Build history of the part. All positions in model axes, mm. Give positions to 0.01 mm unless a question says otherwise; leave off trailing zeros. Loops run counter-clockwise (first coordinate to the right, second up) from the corner with the lowest first, then second, coordinate; pieces in that order, holes last. Notation, with made-up numbers: M 85.25,-27.75 L 143.25,-27.75 A17 cw 143.25,-23.75 Z; hole C 21,-19 d3. An arc over 180 degrees is marked long. Answer as a JSON object with one key per item and string values. Group by question number.
1. Slice it at A-A (y = 25.4). List the corners of the cut face in (x, z).
2. Mould opens along Y. For faces 1 (the face through (0, 1, 6.35)), 2 (the face through (-23.41, 61.62, 3.22)), 3 (the face through (-13.5, 56.4, 3.2)) say: released by +Y, released by -Y, zero draft, split by the parting line, or undercut.
3. Slice it at C-C (x = 12.7). List the corners of the cut face in (y, z).
4. Drop a flat-ended pin along its axis: pin 1 Ø3 at (x, y) = (-12.7, 53.975) entering from -Z. Give the stop position or say it passes through.
5. Drill centre lines: line 1 along X through (y, z) = (-38.1, 3.75); line 2 along Y through (x, z) = (-12.7, 3.5); line 3 along Y through (x, z) = (13, 6). Where is each one in solid material? Low to high. Write a range as [from, to].
6. Slice it at B-B (z = 1). List the corners of the cut face in (x, y) (3 decimals), then the cut area to 3 significant figures.
Autodesk Inventor part; units mm, degrees
ref_plane "YZ Plane" through (0, 0, 0) normal (1, 0, 0) x (0, 1, 0)
ref_plane "XZ Plane" through (0, 0, 0) normal (0, 1, 0) x (-1, 0, 0)
ref_plane "XY Plane" through (0, 0, 0) normal (0, 0, 1) x (1, 0, 0)
sketch "Sketch1" plane through (0, 0, 0) normal (0, 0, 1) x (1, 0, 0)
  line L0 (25.4, -63.5) -> (-25.4, -63.5)
  line L1 (-25.4, -63.5) -> (-25.4, 63.5)
  line L2 (-25.4, 63.5) -> (25.4, 63.5)
  line L3 (25.4, 63.5) -> (25.4, -63.5)
  line L4 (25.4, -63.5) -> (-25.4, 63.5) construction
  line L5 (-25.4, -63.5) -> (25.4, 63.5) construction
  line L6 (-12.7, 53.975) -> (12.7, 53.975) construction
  point P0 (0, 0)
  point P1 (-12.7, 25.4)
  point P2 (12.7, 25.4)
  point P3 (12.7, -38.1)
  point P4 (-12.7, -38.1)
  point P5 (0, 53.975)
  point P6 (0, 63.5)
  dimension "d0" = 50.8
  dimension "d1" = 127
  dimension "d2" = 9.525
  dimension "d3" = 25.4
  dimension "d4" = 38.1
  dimension "d5" = 63.5
extrude "Extrusion1" add sketch "Sketch1" along normal blind 6.35
hole "Hole1" at (-12.7, 53.975, 0) at (12.7, 53.975, 0) at (-12.7, 25.4, 0) at (12.7, 25.4, 0) at (12.7, -38.1, 0) at (-12.7, -38.1, 0) direction (0, 0, 1) diameter 5.1054 end through all
fillet "Fillet1" radius 6.604 4 edges at (25.4, 63.5, 3.175) (-25.4, 63.5, 3.175) (25.4, -63.5, 3.175) (-25.4, -63.5, 3.175)
properties part number "CL7-GB-003" material "Polycarbonate, Clear"
Established:
{
 "1": {"outline": "M -25.4,0 L -15.25,0 L -15.25,6.35 L -25.4,6.35 Z; M -10.15,0 L 10.15,0 L 10.15,6.35 L -10.15,6.35 Z; M 15.25,0 L 25.4,0 L 25.4,6.35 L 15.25,6.35 Z"},
 "2": {"face 1": "zero draft", "face 2": "released by +Y", "face 3": "undercut"},
 "3": {"outline": "M -63.5,0 L -40.65,0 L -40.65,6.35 L -63.5,6.35 Z; M -35.55,0 L 22.85,0 L 22.85,6.35 L -35.55,6.35 Z; M 27.95,0 L 51.42,0 L 51.42,6.35 L 27.95,6.35 Z; M 56.53,0 L 63.5,0 L 63.5,6.35 L 56.53,6.35 Z"},
 "4": {"pin 1": "passes through"},
 "5": {"line 1": "x = [-25.4, -15.25], [-10.15, 10.15], [15.25, 25.4]", "line 2": "y = [-63.5, -40.65], [-35.55, 22.85], [27.95, 51.42], [56.53, 63.5]", "line 3": "y = [-63.5, -40.64], [-35.56, 22.86], [27.94, 51.44], [56.51, 63.5]"},
 "6": {"outline": "M -25.4,-56.896 A6.604 ccw -18.796,-63.5 L 18.796,-63.5 A6.604 ccw 25.4,-56.896 L 25.4,56.896 A6.604 ccw 18.796,63.5 L -18.796,63.5 A6.604 ccw -25.4,56.896 Z; hole C -12.7,-38.1 d5.105; hole C -12.7,25.4 d5.105; hole C -12.7,53.975 d5.105; hole C 12.7,-38.1 d5.105; hole C 12.7,25.4 d5.105; hole C 12.7,53.975 d5.105", "area": "6,290 mm^2"}
}
